Check sheet for the modelled part. Datum: model origin and axes. Units: mm. A direction names the side the tool comes from. Round coordinates to 2 decimals unless told otherwise and drop trailing zeros. Order: outer loops, then holes, each group sorted by start corner. A loop starts at its lowest first (then second) coordinate and runs counter-clockwise, first axis right, second up. Notation, with made-up numbers: (-2, -2) -> (54, -2) arc R22 cw to (54, 11) -> close; hole circle Ø8 at (-34, -36). An arc over 180 degrees is marked (long way). Answer in a Markdown table with one row per item.
```python
from build123d import *
from build123d.topology import SkipClean

# Parameters (mm, degrees)
BOSS_EXTRUDE1_DEPTH             = 14
SKETCH2_R                       = 2.5
CUT_EXTRUDE1_DEPTH              = 31.004166377
SKETCH3_R                       = 9.5
CUT_EXTRUDE2_DEPTH              = 2
CUT_EXTRUDE3_START              = 8
SKETCH3_2_R                     = 9.5
CUT_EXTRUDE3_DEPTH              = 2
BOSS_EXTRUDE2_REACH             = 26.8
BOSS_EXTRUDE2_DIRECTION_2_REACH = 26.8
SKETCH5_R                       = 1.75
CUT_EXTRUDE4_DEPTH              = 3.6
CUT_EXTRUDE5_DEPTH              = 3.5
SKETCH7_R                       = 4.9
CUT_EXTRUDE6_DEPTH              = 1
SKETCH9_R                       = 3.5
SKETCH9_R_2                     = 2.5
BOSS_EXTRUDE3_DEPTH             = 0.3
BOSS_EXTRUDE5_START             = 9.8
SKETCH9_2_R                     = 3.5
SKETCH9_2_R_2                   = 2.5
BOSS_EXTRUDE5_DEPTH             = 0.2
FILLET1_R                       = 4
CHAMFER1_SIZE                   = 0.5
CHAMFER2_SIZE                   = 0.3
CHAMFER3_SIZE                   = 0.5


with BuildPart() as part:
    # Sketch1 → Boss-Extrude1 (new body)
    with BuildSketch(Plane.XY):
        Polygon((0, -9.75), (18, -9.75), (18, 9.75), (0, 9.75), (0, 5), (13, 5), (13, -5), (0, -5), align=None)
    extrude(amount=BOSS_EXTRUDE1_DEPTH)

    # Sketch2 → Cut-Extrude1 (cut, through all)
    with BuildSketch(Plane(origin=(0, 9.75, 0), x_dir=(1, 0, 0), z_dir=(0, 1, 0))):
        with Locations(Location((6, -7, 0), (0, 0, 180))):
            Circle(SKETCH2_R)
    extrude(amount=-CUT_EXTRUDE1_DEPTH, mode=Mode.SUBTRACT)

    # Sketch3 → Cut-Extrude2 (cut)
    with BuildSketch(Plane(origin=(0, -5, 0), x_dir=(1, 0, 0), z_dir=(0, 1, 0))):
        with Locations((6, -7)):
            Circle(SKETCH3_R)
    extrude(amount=CUT_EXTRUDE2_DEPTH, mode=Mode.SUBTRACT)

    # Sketch3<2> → Cut-Extrude3 (cut)
    with BuildSketch(Plane(origin=(0, -5, 0), x_dir=(1, 0, 0), z_dir=(0, 1, 0)).offset(CUT_EXTRUDE3_START)):
        with Locations((6, -7)):
            Circle(SKETCH3_2_R)
    extrude(amount=CUT_EXTRUDE3_DEPTH, mode=Mode.SUBTRACT)

    # Boss-Extrude2: up to this face of the body (flat: up to its plane)
    boss_extrude2_end = Plane(part.part.faces().sort_by_distance((14.012212464, 3, 7))[0])
    # Sketch4 → Boss-Extrude2 (add, up to the picked face)
    with BuildSketch(Plane(origin=(0, 0, 0), x_dir=(1, 0, 0), z_dir=(0, 1, 0)), mode=Mode.PRIVATE) as boss_extrude2_sk1:
        with BuildLine():
            Line((10, -14), (13.722333535, -14))
            Line((13.722333535, -14), (13.722333535, 0))
            Line((13.722333535, 0), (10, 0))
            Line((10, 0), (10, -1.255437353))
            ThreePointArc((10, -1.255437353), (13, -7), (10, -12.744562647))
            Line((10, -12.744562647), (10, -14))
        make_face()
    boss_extrude2_tool1 = split(extrude(boss_extrude2_sk1.sketch, amount=BOSS_EXTRUDE2_REACH, mode=Mode.PRIVATE), bisect_by=boss_extrude2_end, keep=Keep.BOTH, mode=Mode.PRIVATE)
    add(boss_extrude2_tool1.solids().sort_by(Axis((10.144864, 0, 13.372281), (0, 1, 0)))[0])

    # Boss-Extrude2 direction 2: up to this face of the body (flat: up to its plane)
    boss_extrude2_direction_2_end = Plane(part.part.faces().sort_by_distance((14.012212464, -3, 7))[0])
    # Sketch4 → Boss-Extrude2 direction 2 (add, up to the picked face)
    with BuildSketch(Plane(origin=(0, 0, 0), x_dir=(1, 0, 0), z_dir=(0, 1, 0)), mode=Mode.PRIVATE) as boss_extrude2_direction_2_sk1:
        with BuildLine():
            Line((10, -14), (13.722333535, -14))
            Line((13.722333535, -14), (13.722333535, 0))
            Line((13.722333535, 0), (10, 0))
            Line((10, 0), (10, -1.255437353))
            ThreePointArc((10, -1.255437353), (13, -7), (10, -12.744562647))
            Line((10, -12.744562647), (10, -14))
        make_face()
    boss_extrude2_direction_2_tool1 = split(extrude(boss_extrude2_direction_2_sk1.sketch, amount=-BOSS_EXTRUDE2_DIRECTION_2_REACH, mode=Mode.PRIVATE), bisect_by=boss_extrude2_direction_2_end, keep=Keep.BOTH, mode=Mode.PRIVATE)
    add(boss_extrude2_direction_2_tool1.solids().sort_by(Axis((10.144864, 0, 13.372281), (0, -1, 0)))[0])

    # Sketch5 → Cut-Extrude4 (cut)
    with BuildSketch(Plane(origin=(18, 0, 0), x_dir=(0, 0, -1), z_dir=(1, 0, 0))):
        with Locations(Location((-7, 0, 0), (0, 0, 90))):
            Circle(SKETCH5_R)
    extrude(amount=-CUT_EXTRUDE4_DEPTH, mode=Mode.SUBTRACT)

    # Sketch6 → Cut-Extrude5 (cut)
    with BuildSketch(Plane(origin=(0, 9.75, 0), x_dir=(1, 0, 0), z_dir=(0, 1, 0))):
        Polygon((6, -2.381197846), (2, -4.690598923), (2, -9.309401077), (6, -11.618802154), (10, -9.309401077), (10, -4.690598923), align=None)
    extrude(amount=-CUT_EXTRUDE5_DEPTH, mode=Mode.SUBTRACT)

    # Sketch7 → Cut-Extrude6 (cut)
    with BuildSketch(Plane.XZ.offset(9.75)):
        with Locations(Location((6, 7, 0), (0, 0, 270))):
            Circle(SKETCH7_R)
    extrude(amount=-CUT_EXTRUDE6_DEPTH, mode=Mode.SUBTRACT)

    # Sketch9 → Boss-Extrude3 (add)
    with SkipClean():  # the faces are left unmerged after this step: merging them gives an invalid solid
        with BuildSketch(Plane.XZ.offset(-5)):
            with Locations(Location((6, 7, 0), (0, 0, 90))):
                Circle(SKETCH9_R)
            with Locations(Location((6, 7, 0), (0, 0, 270))):
                Circle(SKETCH9_R_2, mode=Mode.SUBTRACT)
        extrude(amount=BOSS_EXTRUDE3_DEPTH)

    # Sketch9<2> → Boss-Extrude5 (add)
    with SkipClean():  # the faces are left unmerged after this step: merging them gives an invalid solid
        with BuildSketch(Plane.XZ.offset(-5).offset(BOSS_EXTRUDE5_START)):
            with Locations(Location((6, 7, 0), (0, 0, 90))):
                Circle(SKETCH9_2_R)
            with Locations(Location((6, 7, 0), (0, 0, 270))):
                Circle(SKETCH9_2_R_2, mode=Mode.SUBTRACT)
        extrude(amount=BOSS_EXTRUDE5_DEPTH)

    # Fillet1
    fillet1_edges = [part.edges().sort_by_distance(p)[0] for p in [
        (0, -7.375, 0),
        (18, 0, 14),
        (0, 7.375, 0),
    ]]
    fillet(fillet1_edges, radius=FILLET1_R)

    # Chamfer1
    chamfer1_edges = [part.edges().sort_by_distance(p)[0] for p in [
        (8, 9.75, 3.535898385),
        (4, 9.75, 3.535898385),
        (2, 9.75, 7),
        (4, 9.75, 10.464101615),
        (8, 9.75, 10.464101615),
        (10, 9.75, 7),
        (6, -9.75, 11.9),
    ]]
    chamfer(chamfer1_edges, length=CHAMFER1_SIZE)

    # Chamfer2
    # the kernel refuses this chamfer: 0.3 mm, written as the material it takes off along each edge
    with BuildSketch(Plane(origin=(6, 4.7, 7), x_dir=(0, 0, 1), z_dir=(1, 0, 0))) as chamfer2_piece_1_section:
        Polygon((3.5, -CHAMFER2_SIZE), (3.5 - CHAMFER2_SIZE, 0), (3.5, 0), align=None)
    chamfer2_piece_1 = revolve(axis=Axis((6, 4.7, 7), (0, -1, 0)), mode=Mode.PRIVATE)
    chamfer2_piece_1 = split(chamfer2_piece_1, bisect_by=Plane(origin=(6, 5, 3.647041133), z_dir=(0, -1, 0)), keep=Keep.TOP, mode=Mode.PRIVATE)
    add(chamfer2_piece_1, mode=Mode.SUBTRACT)
    with BuildSketch(Plane(origin=(6, -4.8, 7), x_dir=(0, 0, 1), z_dir=(1, 0, 0))) as chamfer2_piece_2_section:
        Polygon((3.5, CHAMFER2_SIZE), (3.5 - CHAMFER2_SIZE, 0), (3.5, 0), align=None)
    chamfer2_piece_2 = revolve(axis=Axis((6, -4.8, 7), (0, -1, 0)), mode=Mode.PRIVATE)
    chamfer2_piece_2 = split(chamfer2_piece_2, bisect_by=Plane(origin=(6, -5, 3.697354153), z_dir=(0, 1, 0)), keep=Keep.TOP, mode=Mode.PRIVATE)
    add(chamfer2_piece_2, mode=Mode.SUBTRACT)

    # Chamfer3
    chamfer3_edges = [part.edges().sort_by_distance(p)[0] for p in [
        (11, 9.75, 0),
        (18, 0, 0),
        (8.5, 6.25, 7),
        (8.5, -8.75, 7),
        (0, -5, 9),
        (0, 5, 9),
        (0, 9.75, 9),
        (0, -9.75, 9),
        (11, -9.75, 0),
        (18, -9.75, 5),
        (16.828427125, -9.75, 12.828427125),
        (1.171572875, -9.75, 1.171572875),
        (8.5, 5, 0),
        (1.171572875, -5, 1.171572875),
        (1.171572875, 5, 1.171572875),
        (7, 9.75, 14),
        (18, 9.75, 5),
        (16.828427125, 9.75, 12.828427125),
        (1.171572875, 9.75, 1.171572875),
        (0, 7.375, 14),
        (6.5, 5, 14),
        (6.5, -5, 14),
        (0, -7.375, 14),
        (10, 0, 14),
        (11.5, -3, 14),
        (11.5, 3, 0),
        (11.5, 3, 14),
        (10, 0, 0),
        (11.5, -3, 0),
        (8.5, -5, 0),
        (7, -9.75, 14),
    ]]
    chamfer(chamfer3_edges, length=CHAMFER3_SIZE)


solid = part.part
```
(1) Section check A-A on y = -6. Record the boundary of the cut face in (x, z), plus the area to 3 significant figures.
Solutions:
| item | result |
|---|---|
| outline | (0, 4) arc R4 ccw to (4, 0) -> (17.5, 0) -> (18, 0.5) -> (18, 10) arc R4 ccw to (14, 14) -> (0.5, 14) -> (0, 13.5) -> close; hole circle Ø5 at (6, 7) |
| area | 225 mm^2 |
(2) Draft check along X on faces 1 (the flat face through (10, 5, 7)), 2 (the cylindrical face through (13, 0, 7)), 3 (the cylindrical face through (4.123, -9.004, 2.474)), 4 (the flat face through (14.4, 0, 7)). Enter one of: pulls with the +X half, pulls with the -X half, needs draft (parallel to the pull), parting line crosses it, or undercut.
Solutions:
| item | result |
|---|---|
| face 1 | undercut |
| face 2 | pulls with the -X half |
| face 3 | undercut |
| face 4 | pulls with the +X half |
(3) Depth check by flat-ended pin: pin 1 Ø5 at (y, z) = (-1.5, 7.5) entering from -X; pin 2 Ø5 at (x, z) = (5, 6.5) entering from -Y; pin 3 Ø1.5 at (x, z) = (2.5, 5) entering from +Y; pin 4 Ø8 at (x, y) = (3, 3.5) entering from -Z. Enter the tip coordinate at first touch or a pass-through.
Solutions:
| item | result |
|---|---|
| pin 1 | x = 12.32 |
| pin 2 | y = -8.75 |
| pin 3 | y = 9.5 |
| pin 4 | z = 0 |
(4) Tool access check on faces 5 (the flat face through (13.3, 3, 6.9)), 6 (the conical face through (1.458, -5.135, 1.401)), 7 (the flat face through (7.97, 7.77, 10.48)), 8 (the cylindrical face through (16.23, -0.38, 5.29)). Record the directions out of +Z, -Z, +X, -X, +Y, -Y that give a thin tool (end or side, any length) a straight path to the whole face; none if there is none.
Solutions:
| item | result |
|---|---|
| face 5 | -X |
| face 6 | -Z, -X |
| face 7 | +Y |
| face 8 | +X |
(5) Section check B-B on y = 4. Record the boundary of the cut face in (x, z).
Solutions:
| item | result |
|---|---|
| outline | (13, 0) -> (17.5, 0) -> (18, 0.5) -> (18, 10) arc R4 ccw to (14, 14) -> (13, 14) -> (13, 13.42) arc R9.5 cw to (13, 0.58) -> close |
(6) Scan lines: probe 1 along Y at (x, z) = (13.5, 8.5); probe 2 along Z at (x, y) = (6, 5.65); probe 3 along Y at (x, z) = (2.5, 10). Record each from-to range of solid material in increasing order. Write a range as from..to.
Solutions:
| item | result |
|---|---|
| probe 1 | -9.75..-5, -3..3, 5..9.75 |
| probe 2 | 0..4.5, 9.5..14 |
| probe 3 | -8.75..-5, 5..9.6 |
(7) Section check C-C on z = 7. Give the number of separate pieces and of enclosed holes in the cut face, plus the area to 3 significant figures.
Solutions:
| item | result |
|---|---|
| separate pieces | 3 |
| enclosed holes | 0 |
| area | 135 mm^2 |
(8) Section check D-D on y = 0. Record the boundary of the cut face in (x, z).
Solutions:
| item | result |
|---|---|
| outline | (10, 0.5) -> (10.5, 0) -> (17.5, 0) -> (18, 0.5) -> (18, 5.25) -> (14.4, 5.25) -> (14.4, 8.75) -> (18, 8.75) -> (18, 10) arc R4 ccw to (14, 14) -> (10.5, 14) -> (10, 13.5) -> (10, 12.74) arc R7 cw to (10, 1.26) -> close |
